```python
from build123d import *
from build123d import SkipClean  # not in build123d's __all__

# Parameters (mm, degrees)
F0_R     = 1.5
F1_DEPTH = 4
F2_R     = 0.55
F3_R     = 1
F4_R     = 0.5499
F6_DEPTH = 5.5


# Not quite as in the source:
# - a fillet or chamfer is up to 0.001 mm smaller than in the source, because OpenCascade refuses the exact size
# - a feature names something its author has since deleted; it is built from what else it names


with BuildPart() as f1:
    # F0 (on Top) → F1 (new body)
    with BuildSketch(Plane.XY):
        with BuildLine():
            Line((-95, 0), (0, 0))
            ThreePointArc((0, 0), (3, -3), (6, 0))
            Line((6, 0), (13, 0))
            ThreePointArc((13, 0), (16.5355339059, 1.4644660941), (18, 5))
            Line((18, 5), (18, 10))
            ThreePointArc((18, 10), (16.5355339059, 13.5355339059), (13, 15))
            Line((13, 15), (6, 15))
            ThreePointArc((6, 15), (3, 18), (0, 15))
            Line((0, 15), (-95, 15))
            ThreePointArc((-95, 15), (-98.5355339059, 13.5355339059), (-100, 10))
            Line((-100, 10), (-100, 5))
            ThreePointArc((-100, 5), (-98.5355339059, 1.4644660941), (-95, 0))
        make_face()
        with Locations((3, 0)):
            Circle(F0_R, mode=Mode.SUBTRACT)
        with Locations((3, 15)):
            Circle(F0_R, mode=Mode.SUBTRACT)
    extrude(amount=F1_DEPTH)

    # F2
    f2_edges = [f1.edges().sort_by_distance(p)[0] for p in [
        (-47.5, 0, 4),
    ]]
    fillet(f2_edges, radius=F2_R)

    # F3
    f3_edges = [f1.edges().sort_by_distance(p)[0] for p in [
        (-47.5, 0, 0),
    ]]
    fillet(f3_edges, radius=F3_R)

    # F4 (radius 0.55 in the source; OpenCascade refuses exactly that, so slightly less here)
    f4_edges = [f1.edges().sort_by_distance(p)[0] for p in [
        (3, 18, 4),
        (3, 18, 0),
        (9.5, 0, 4),
        (16.535534, 13.535534, 4),
        (16.535534, 1.464466, 4),
        (16.535534, 13.535534, 0),
        (16.535534, 1.464466, 0),
        (9.5, 0, 0),
        (9.5, 15, 0),
        (9.5, 15, 4),
    ]]
    fillet(f4_edges, radius=F4_R)

    # F5 (on Top) → F6 (join)
    with BuildSketch(Plane.XY):
        with BuildLine():
            Line((12.9997539334, 8.5000049546), (-6.9997087121, 8.5000049546))
            ThreePointArc((-6.9997087121, 8.5000049546), (-7.9997087121, 7.5000049546), (-6.9997087121, 6.5000049546))
            Line((-6.9997087121, 6.5000049546), (12.9997539334, 6.5000049546))
            ThreePointArc((12.9997539334, 6.5000049546), (13.9997539334, 7.5000049546), (12.9997539334, 8.5000049546))
        make_face()
    with SkipClean():  # cleaning this boolean's faces spoils the solid; the shape is the same uncleaned
        extrude(amount=F6_DEPTH)


solid = f1.part
```
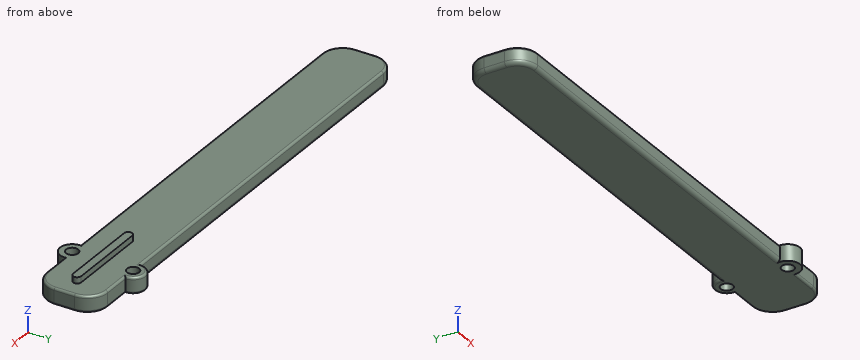
Work out the finished part from the listing and answer in its coordinate system (mm). Coordinates: 2 decimals unless noted, no trailing zeros. Loops run counter-clockwise (first coordinate to the right, second up) from the corner with the lowest first, then second, coordinate; pieces in that order, holes last. Notation, with made-up numbers: (43.25, 2) - (69.25, 2) arc R37 cw to (69.25, 41) - close; hole circle Ø10 at (8, 59). An arc over 180 degrees is marked (long way). Use a Markdown table: item, result.
Item 1: Given pin 1 Ø5 at (x, y) = (-86.5, 3) entering from +Z; pin 2 Ø1.6 at (x, z) = (0, 5) entering from -Y; pin 3 Ø0.9 at (x, z) = (8, 1.5) entering from -Y; pin 4 Ø2.5 at (x, y) = (3, 0) entering from -Z, each flat-ended and moving along its own axis, determine where each tip first touches the part or whether it passes through.
Evaluation:
| item | result |
|---|---|
| pin 1 | stops at z = 4 |
| pin 2 | stops at y = 6.5 |
| pin 3 | stops at y = 0 |
| pin 4 | passes through |
Item 2: Consider probe 1 along Y at (x, z) = (3, 1.15); probe 2 along Z at (x, y) = (-18.5, 14); probe 3 along Y at (x, z) = (-45, 3.05). Determine where each line is inside the solid, lowest interval first. Write a range as from..to.
Evaluation:
| item | result |
|---|---|
| probe 1 | y = -3..-1.5, 1.5..13.5, 16.5..18 |
| probe 2 | z = 0..4 |
| probe 3 | y = 0..15 |
Item 3: Find section A-A, the plane x = 3. Determine the outline of the cut face in (y, z).
Evaluation:
| item | result |
|---|---|
| outline | (-3, 0) - (-1.5, 0) - (-1.5, 4) - (-3, 4) - close; (1.5, 0) - (13.5, 0) - (13.5, 4) - (8.5, 4) - (8.5, 5.5) - (6.5, 5.5) - (6.5, 4) - (1.5, 4) - close; (16.5, 0) - (17.45, 0) arc R0.55 ccw to (18, 0.55) - (18, 3.45) arc R0.55 ccw to (17.45, 4) - (16.5, 4) - close |
Item 4: Find section B-B, the plane x = -57. Determine the outline of the cut face in (y, z), and give its area (3 significant figures).
Evaluation:
| item | result |
|---|---|
| outline | (0, 1) arc R1 ccw to (1, 0) - (14, 0) arc R1 ccw to (15, 1) - (15, 3.45) arc R0.55 ccw to (14.45, 4) - (0.55, 4) arc R0.55 ccw to (0, 3.45) - close |
| area | 59.4 mm2 |
